```python
from build123d import *

# Parameters (mm, degrees)
BOSS_EXTRUDE1_DEPTH = 8
SKETCH2_R           = 2.4
BOSS_EXTRUDE2_DEPTH = 1.6
SHELL1_START        = -8
SHELL1_OUTLINE_W    = 28.8
SHELL1_OUTLINE_H    = 4.8
SHELL1_DEPTH        = 8
SHELL1_START_2      = -9.6
SHELL1_2_OUTLINE_R  = 0.8
SHELL1_2_DEPTH      = 1.6


# Read off the part's stored shape, not the designer's step: Shell1
with BuildPart() as part:
    # Sketch1 → Boss-Extrude1 (new body)
    with BuildSketch(Plane(origin=(0, 0, 0), x_dir=(1, 0, 0), z_dir=(0, 1, 0))):
        Polygon((-16, 0), (16, 0), (16, 9.6), (14, 9.6), (14, 12.6), (12, 12.6), (12, 9.6), (-12, 9.6), (-12, 12.6), (-14, 12.6), (-14, 9.6), (-16, 9.6), align=None)
    extrude(amount=BOSS_EXTRUDE1_DEPTH)

    # Sketch2 → Boss-Extrude2 (add)
    with BuildSketch(Plane(origin=(0, 0, -9.6), x_dir=(-1, 0, 0), z_dir=(0, 0, -1))):
        with Locations(Location((4, 4, 0), (0, 0, 180))):
            Circle(SKETCH2_R)
        with Locations(Location((-4, 4, 0), (0, 0, 180))):
            Circle(SKETCH2_R)
    extrude(amount=BOSS_EXTRUDE2_DEPTH)

    # Shell1 outline → Shell1 (cut)
    with BuildSketch(Plane.XY.offset(SHELL1_START)):
        with Locations((0, 4)):
            Rectangle(SHELL1_OUTLINE_W, SHELL1_OUTLINE_H)
    extrude(amount=SHELL1_DEPTH, mode=Mode.SUBTRACT)

    # Shell1 2 outline → Shell1 2 (cut)
    with BuildSketch(Plane.XY.offset(SHELL1_START_2)):
        with Locations((-4, 4)):
            Circle(SHELL1_2_OUTLINE_R)
        with Locations((4, 4)):
            Circle(SHELL1_2_OUTLINE_R)
    extrude(amount=SHELL1_2_DEPTH, mode=Mode.SUBTRACT)


solid = part.part
```
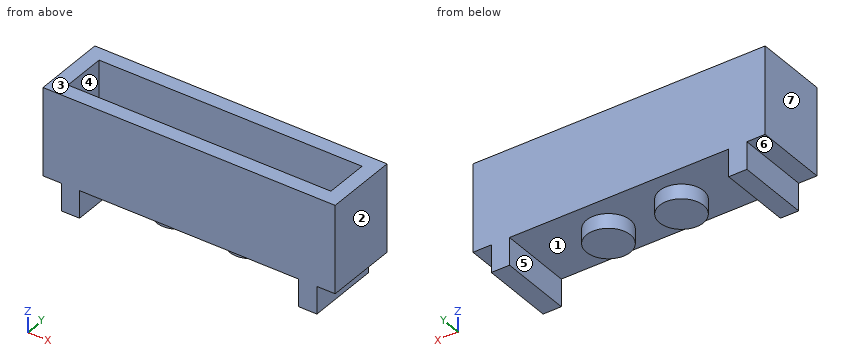
Geometry check sheet. Reference: the model listing, model coordinates, mm. Face numbers are marked on the shaded views. A direction names the side the tool comes from. Round coordinates to 2 decimals unless told otherwise and drop trailing zeros. Loops run counter-clockwise (first coordinate to the right, second up) from the corner with the lowest first, then second, coordinate; pieces in that order, holes last. Notation, with made-up numbers: (79.25, 16.25) - (83.25, 16.25) arc R17 cw to (83.25, 38.25) - close; hole circle Ø7 at (-17.75, -4.75). An arc over 180 degrees is marked (long way). Write each question's results on one line, items separated by ' | '. Start each with the question number.
Q1. Thickness scan on line 1 (X direction, y = 4, z = -10.5); line 2 (Y direction, x = 0, z = -5.25); line 3 (Y direction, x = -4, z = -8.4). Record the ranges inside material, lowest first. Write a range as [from, to].
Q2. Cross-section at C-C on x = 4. Enter the section's corners in (y, z).
Q3. Access from +Z, -Z, +X, -X, +Y, -Y to the whole of each face (thin tool, end or side, straight path). Record for the marked faces 4, 5, 6 and 7.
Q4. Release check for a two-part mould opening along X. For the marked faces 1, 2 and 3 record: +X half, -X half, draft (parallel to the pull), parting line (faces both ways), or undercut.
Q5. Gauge pin test, flat ends, axial feed: P1, Ø2, axis at x = 14.5, y = 3, coming from the -Z side; P2, Ø4, axis at x = 3.5, y = 4.5, coming from the -Z side; P3, Ø1.5, axis at y = 4, z = -10.5, coming from the -X side; P4, Ø1.5, axis at y = 2.5, z = -11.5, coming from the +X side. Record the tip position at first contact, or that the pin passes through.
Q6. Cross-section at D-D on x = 8.5. Enter the section's corners in (y, z), and give its area (3 significant figures).
Q7. Cross-section at B-B on z = -2.5. Enter the section's corners in (x, y), and give its area (3 significant figures).
Answers below:
1) line 1: x = [-14, -12], [-6.4, -1.6], [1.6, 6.4], [12, 14] | line 2: y = [0, 1.6], [6.4, 8] | line 3: y = [0, 3.2], [4.8, 8]
2) outline: (0, -9.6) - (1.6, -9.6) - (1.6, -11.2) - (6.4, -11.2) - (6.4, -9.6) - (8, -9.6) - (8, 0) - (6.4, 0) - (6.4, -8) - (4.8, -8) - (4.8, -9.6) - (3.2, -9.6) - (3.2, -8) - (1.6, -8) - (1.6, 0) - (0, 0) - close
3) face 4: +Z | face 5: -Z, +Y, -Y | face 6: -Z, -X, +Y, -Y | face 7: +Z, -Z, -X, +Y, -Y
4) face 1: undercut | face 2: +X half | face 3: draft
5) P1: stops at z = -12.6 | P2: stops at z = -11.2 | P3: stops at x = -14 | P4: stops at x = 14
6) outline: (0, -9.6) - (8, -9.6) - (8, 0) - (6.4, 0) - (6.4, -8) - (1.6, -8) - (1.6, 0) - (0, 0) - close | area: 38.4 mm²
7) outline: (-16, 0) - (16, 0) - (16, 8) - (-16, 8) - close; hole (-14.4, 1.6) - (14.4, 1.6) - (14.4, 6.4) - (-14.4, 6.4) - close | area: 118 mm²
